from build123d import *

# Parameters (mm, degrees)
SKETCH2_W           = 25.4
SKETCH2_H           = 50.8
SKETCH2_R           = 3.5
BOSS_EXTRUDE4_DEPTH = 4
BOSS_EXTRUDE5_START = 4
BOSS_EXTRUDE5_DEPTH = 90
CUT_EXTRUDE2_START  = 8
SKETCH2_6_W         = 11.5
SKETCH2_6_H         = 13
CUT_EXTRUDE2_DEPTH  = 6
SKETCH2_7_R         = 3.5
CUT_EXTRUDE3_DEPTH  = 25
BOSS_EXTRUDE6_DEPTH = 4
FILLET1_R           = 4


with BuildPart() as part:
    # Sketch2 → Boss-Extrude4 (new body)
    with BuildSketch(Plane.XY):
        Rectangle(SKETCH2_W, SKETCH2_H)
        with Locations((0, 12.7)):
            Circle(SKETCH2_R, mode=Mode.SUBTRACT)
        with Locations((0, -12.7)):
            Circle(SKETCH2_R, mode=Mode.SUBTRACT)
    extrude(amount=BOSS_EXTRUDE4_DEPTH)

    # Sketch2<4> → Boss-Extrude5 (add)
    with BuildSketch(Plane.XY.offset(BOSS_EXTRUDE5_START)):
        with BuildLine():
            Line((12.7, -12.7), (5.75, -12.7))
            Line((5.75, -12.7), (5.75, -19.2))
            Line((5.75, -19.2), (-5.75, -19.2))
            Line((-5.75, -19.2), (-5.75, -12.7))
            Line((-5.75, -12.7), (-12.7, -12.7))
            Line((-12.7, -12.7), (-12.7, -18.208514492))
            ThreePointArc((-12.7, -18.208514492), (0, -22.2), (12.7, -18.208514492))
            Line((12.7, -18.208514492), (12.7, -12.7))
        make_face()
        with BuildLine():
            Line((5.75, -19.2), (5.75, -12.7))
            Line((5.75, -12.7), (3.5, -12.7))
            ThreePointArc((3.5, -12.7), (0, -16.2), (-3.5, -12.7))
            Line((-3.5, -12.7), (-5.75, -12.7))
            Line((-5.75, -12.7), (-5.75, -19.2))
            Line((-5.75, -19.2), (5.75, -19.2))
        make_face()
        with BuildLine():
            Line((5.75, -12.7), (5.75, -6.2))
            Line((5.75, -6.2), (-5.75, -6.2))
            Line((-5.75, -6.2), (-5.75, -12.7))
            Line((-5.75, -12.7), (-3.5, -12.7))
            ThreePointArc((-3.5, -12.7), (0, -9.2), (3.5, -12.7))
            Line((3.5, -12.7), (5.75, -12.7))
        make_face()
        with BuildLine():
            ThreePointArc((-3.5, -12.7), (0, -16.2), (3.5, -12.7))
            Line((3.5, -12.7), (-3.5, -12.7))
        make_face()
        with BuildLine():
            Line((-3.5, -12.7), (3.5, -12.7))
            ThreePointArc((3.5, -12.7), (0, -9.2), (-3.5, -12.7))
        make_face()
        with BuildLine():
            ThreePointArc((-3.5, 12.7), (0, 9.2), (3.5, 12.7))
            Line((3.5, 12.7), (-3.5, 12.7))
        make_face()
        with BuildLine():
            Line((-3.5, 12.7), (3.5, 12.7))
            ThreePointArc((3.5, 12.7), (0, 16.2), (-3.5, 12.7))
        make_face()
        with BuildLine():
            Line((3.5, 12.7), (5.75, 12.7))
            Line((5.75, 12.7), (5.75, 19.2))
            Line((5.75, 19.2), (-5.75, 19.2))
            Line((-5.75, 19.2), (-5.75, 12.7))
            Line((-5.75, 12.7), (-3.5, 12.7))
            ThreePointArc((-3.5, 12.7), (0, 16.2), (3.5, 12.7))
        make_face()
        with BuildLine():
            Line((5.75, 6.2), (5.75, 12.7))
            Line((5.75, 12.7), (3.5, 12.7))
            ThreePointArc((3.5, 12.7), (0, 9.2), (-3.5, 12.7))
            Line((-3.5, 12.7), (-5.75, 12.7))
            Line((-5.75, 12.7), (-5.75, 6.2))
            Line((-5.75, 6.2), (5.75, 6.2))
        make_face()
        Polygon((-5.75, -6.2), (5.75, -6.2), (5.75, -12.7), (12.7, -12.7), (12.7, 12.7), (5.75, 12.7), (5.75, 6.2), (-5.75, 6.2), (-5.75, 12.7), (-12.7, 12.7), (-12.7, -12.7), (-5.75, -12.7), align=None)
        with BuildLine():
            Line((5.75, 12.7), (12.7, 12.7))
            Line((12.7, 12.7), (12.7, 18.208514492))
            ThreePointArc((12.7, 18.208514492), (0, 22.2), (-12.7, 18.208514492))
            Line((-12.7, 18.208514492), (-12.7, 12.7))
            Line((-12.7, 12.7), (-5.75, 12.7))
            Line((-5.75, 12.7), (-5.75, 19.2))
            Line((-5.75, 19.2), (5.75, 19.2))
            Line((5.75, 19.2), (5.75, 12.7))
        make_face()
    extrude(amount=BOSS_EXTRUDE5_DEPTH)

    # Sketch2<6> → Cut-Extrude2 (cut)
    with BuildSketch(Plane.XY.offset(CUT_EXTRUDE2_START)):
        with Locations((0, -12.7)):
            Rectangle(SKETCH2_6_W, SKETCH2_6_H)
        with Locations((0, 12.7)):
            Rectangle(SKETCH2_6_W, SKETCH2_6_H)
    extrude(amount=CUT_EXTRUDE2_DEPTH, mode=Mode.SUBTRACT)

    # Sketch2<7> → Cut-Extrude3 (cut)
    with BuildSketch(Plane.XY):
        with Locations((0, 12.7)):
            Circle(SKETCH2_7_R)
        with Locations((0, -12.7)):
            Circle(SKETCH2_7_R)
    extrude(amount=CUT_EXTRUDE3_DEPTH, mode=Mode.SUBTRACT)

    # Sketch3 → Boss-Extrude6 (add)
    with BuildSketch(Plane.XY.offset(94)):
        with BuildLine():
            Line((12.7, -18.208514492), (12.7, -26.208514492))
            ThreePointArc((12.7, -26.208514492), (0, -29.123465314), (-12.7, -26.208514492))
            Line((-12.7, -26.208514492), (-12.7, -18.208514492))
            Line((-12.7, -18.208514492), (-12.7, 18.208514492))
            ThreePointArc((-12.7, 18.208514492), (0, 22.2), (12.7, 18.208514492))
            Line((12.7, 18.208514492), (12.7, -18.208514492))
        make_face()
    extrude(amount=BOSS_EXTRUDE6_DEPTH)

    # Fillet1
    fillet1_edges = [part.edges().sort_by_distance(p)[0] for p in [
        (12.7, -26.208514492, 96),
        (-12.7, -26.208514492, 96),
    ]]
    fillet(fillet1_edges, radius=FILLET1_R)


solid = part.part
Design review of the part built by this model. Coordinates are the model's own, in mm. A direction names the side the tool comes from. Coordinates: 2 decimals unless noted, no trailing zeros. Order: outer loops, then holes, each group sorted by start corner. A loop starts at its lowest first (then second) coordinate and runs counter-clockwise, first axis right, second up.
Item 1: Take a section at B-B, the plane z = 6. Write out the cut boundary in (x, y), then the cut area to 3 significant figures.
Item 2: Take a section at D-D, the plane z = 41. Write out the cut boundary in (x, y), then the cut area to 3 significant figures.
Item 3: For pin 1 Ø1.8 at (x, z) = (-2, 11.5) entering from -Y; pin 2 Ø6.5 at (x, z) = (0.5, 10.5) entering from +Y; pin 3 Ø4 at (x, y) = (0, 12.7) entering from -Z, all flat-tipped, find the tip position at first contact; note any pin that passes through.
Item 4: For line 1 (Y direction, x = 0, z = 14.5); line 2 (Y direction, x = 0, z = 3.75); line 3 (X direction, y = -10.5, z = 12), list the stretches that pass through material, from the lowest coordinate up.
Item 5: The part is to be moulded in two halves that separate along X. For faces 1 (the flat face through (12.7, 0, 48)), 2 (the flat face through (-4, -13, 14)), 3 (the flat face through (0, -23, 4)), say which applies: pulls with the +X half, pulls with the -X half, needs draft (parallel to the pull), parting line crosses it, or undercut.
Item 6: For faces 4 (the cylindrical face through (1.88, -9.75, 19.42)), 5 (the cylindrical face through (11.962, -25.884, 96.028)), 6 (the flat face through (-5.75, -13, 11)), list the 3-axis set-ups (+Z, -Z, +X, -X, +Y, -Y) from which the entire face can be reached by the end or side of a thin tool; tool diameter is ignored.
Item 7: Take a section at C-C, the plane y = -12.7. Write out the cut boundary in (x, z).
The answers:
1. outline: (-12.7, -18.21) arc R22.2 ccw to (12.7, -18.21) - (12.7, 18.21) arc R22.2 ccw to (-12.7, 18.21) - close; hole circle Ø7 at (0, -12.7); hole circle Ø7 at (0, 12.7)
1. area: 986 mm2
2. outline: (-12.7, -18.21) arc R22.2 ccw to (12.7, -18.21) - (12.7, 18.21) arc R22.2 ccw to (-12.7, 18.21) - close
2. area: 1,060 mm2
3. pin 1: stops at y = -22.17
3. pin 2: stops at y = 22.2
3. pin 3: stops at z = 25
4. line 1: y = -22.2 to -16.2, -9.2 to 9.2, 16.2 to 22.2
4. line 2: y = -25.4 to -16.2, -9.2 to 9.2, 16.2 to 25.4
4. line 3: x = -12.7 to -5.75, 5.75 to 12.7
5. face 1: pulls with the +X half
5. face 2: undercut
5. face 3: needs draft
6. face 4: -Z
6. face 5: +Z, +X, -Y
6. face 6: none
7. outline: (-12.7, 0) - (-3.5, 0) - (-3.5, 8) - (-5.75, 8) - (-5.75, 14) - (-3.5, 14) - (-3.5, 25) - (3.5, 25) - (3.5, 14) - (5.75, 14) - (5.75, 8) - (3.5, 8) - (3.5, 0) - (12.7, 0) - (12.7, 98) - (-12.7, 98) - close
